from build123d import *

# Parameters (mm, degrees)
BOSS_EXTRUDE1_START = -1.6129
SKETCH2_W           = 8.89
SKETCH2_H           = 8.89
BOSS_EXTRUDE1_DEPTH = 5.1054
SKETCH3_W           = 1.2446
SKETCH3_H           = 8.89
CUT_EXTRUDE1_DEPTH  = 8.1912173
FILLET1_R           = 0.2794


with BuildPart() as part:
    # Sketch2 → Boss-Extrude1 (new body)
    with BuildSketch(Plane(origin=(0, 0, 0), x_dir=(1, 0, 0), z_dir=(0, 1, 0)).offset(BOSS_EXTRUDE1_START)):
        Rectangle(SKETCH2_W, SKETCH2_H)
    extrude(amount=BOSS_EXTRUDE1_DEPTH)

    # Sketch3 → Cut-Extrude1 (cut, through all)
    with BuildSketch(Plane(origin=(0, 0, 0), x_dir=(1, 0, 0), z_dir=(0, 1, 0))):
        with Locations((-3.04038, 0)):
            Rectangle(SKETCH3_W, SKETCH3_H)
        with Locations((-1.01346, 0)):
            Rectangle(SKETCH3_W, SKETCH3_H)
        with Locations((1.01346, 0)):
            Rectangle(SKETCH3_W, SKETCH3_H)
        with Locations((3.04038, 0)):
            Rectangle(SKETCH3_W, SKETCH3_H)
    extrude(amount=CUT_EXTRUDE1_DEPTH, mode=Mode.SUBTRACT)

    # Fillet1
    fillet1_edges = [part.edges().sort_by_distance(p)[0] for p in [
        (-4.445, 3.4925, 0),
        (-2.41808, 3.4925, 0),
        (-3.66268, 0, 0),
        (-3.66268, 3.4925, 0),
        (-2.41808, 0, 0),
        (4.445, 3.4925, 0),
        (-1.63576, 0, 0),
        (-0.39116, 3.4925, 0),
        (-1.63576, 3.4925, 0),
        (-0.39116, 0, 0),
        (0.39116, 0, 0),
        (1.63576, 3.4925, 0),
        (0.39116, 3.4925, 0),
        (1.63576, 0, 0),
        (2.41808, 0, 0),
        (3.66268, 3.4925, 0),
        (2.41808, 3.4925, 0),
        (3.66268, 0, 0),
    ]]
    fillet(fillet1_edges, radius=FILLET1_R)


solid = part.part
Verification items for the finished model (mm, model axes). A direction names the side the tool comes from. Round coordinates to 2 decimals unless told otherwise and drop trailing zeros. Write each loop counter-clockwise with the first axis right and the second up, starting at its lowest first coordinate (ties: lowest second). Pieces come first, ordered by that corner, then holes.
(1) Access from +Z, -Z, +X, -X, +Y, -Y to the whole of each face (thin tool, end or side, straight path). Record for faces 4 (the flat face through (2.418, 2, 0)), 5 (the flat face through (-4.445, 1, 0)).
Returned:
face 4: +Z, -Z, +Y
face 5: +Z, -Z, -X, +Y, -Y
(2) Section check B-B (y = 0.15). Enter the section's corners in (x, z) (3 decimals).
Returned:
outline: (-4.445, -4.445) - (-3.631, -4.445) - (-3.631, 4.445) - (-4.445, 4.445) - close; (-2.45, -4.445) - (-1.604, -4.445) - (-1.604, 4.445) - (-2.45, 4.445) - close; (-0.423, -4.445) - (0.423, -4.445) - (0.423, 4.445) - (-0.423, 4.445) - close; (1.604, -4.445) - (2.45, -4.445) - (2.45, 4.445) - (1.604, 4.445) - close; (3.631, -4.445) - (4.445, -4.445) - (4.445, 4.445) - (3.631, 4.445) - close
(3) Section check A-A (y = 1.55). Enter the section's corners in (x, z) (3 decimals), plus the area to 3 significant figures.
Returned:
outline: (-4.445, -4.445) - (-3.663, -4.445) - (-3.663, 4.445) - (-4.445, 4.445) - close; (-2.418, -4.445) - (-1.636, -4.445) - (-1.636, 4.445) - (-2.418, 4.445) - close; (-0.391, -4.445) - (0.391, -4.445) - (0.391, 4.445) - (-0.391, 4.445) - close; (1.636, -4.445) - (2.418, -4.445) - (2.418, 4.445) - (1.636, 4.445) - close; (3.663, -4.445) - (4.445, -4.445) - (4.445, 4.445) - (3.663, 4.445) - close
area: 34.8 mm2
(4) Depth check by flat-ended pin: pin 1 Ø0.8 at (x, z) = (-1, 1.5) entering from +Y; pin 2 Ø4 at (x, z) = (3.5, 3) entering from +Y. Enter the tip coordinate at first touch or a pass-through.
Returned:
pin 1: stops at y = 0.01
pin 2: stops at y = 3.49
(5) Material ranges on line 1 (X direction, y = 2.3, z = 3.5) (3 decimals); line 2 (Y direction, x = 3, z = 2.25); line 3 (X direction, y = 0.1, z = 2) (3 decimals), recorded low to high.
Returned:
line 1: x = -4.445 to -3.663, -2.418 to -1.636, -0.391 to 0.391, 1.636 to 2.418, 3.663 to 4.445
line 2: y = -1.61 to 0
line 3: x = -4.445 to -3.597, -2.483 to -1.571, -0.456 to 0.456, 1.571 to 2.483, 3.597 to 4.445
(6) Section check D-D (x = -3.5). Enter the section's corners in (y, z) (3 decimals).
Returned:
outline: (-1.613, -4.445) - (0.026, -4.445) - (0.026, 4.445) - (-1.613, 4.445) - close
(7) Section check C-C (x = 3.25). Enter the section's corners in (y, z) (3 decimals).
Returned:
outline: (-1.613, -4.445) - (0, -4.445) - (0, 4.445) - (-1.613, 4.445) - close
(8) Mould release check, pull along X, two halves, no side actions. Record for faces 1 (the flat face through (-1.636, 2, 0)), 2 (the flat face through (0, -1.613, 0)), 3 (the flat face through (4.445, 1, 0)): pulls with the +X half, pulls with the -X half, needs draft (parallel to the pull), parting line crosses it, or undercut.
Returned:
face 1: undercut
face 2: needs draft
face 3: pulls with the +X half
